from build123d import *

# Parameters (mm, degrees)
ESBO_O1_R                = 20
RESSALTO_EXTRUS_O1_DEPTH = 2
ESBO_O2_R                = 6
RESSALTO_EXTRUS_O2_DEPTH = 8
FILETE3_R                = 8
ESBO_O3_R                = 1.55
CORTE_EXTRUS_O1_DEPTH    = 30.393876913
PADR_OCIRCULAR1_COUNT    = 4
ESBO_O5_R                = 3.75
CORTE_EXTRUS_O2_DEPTH    = 6
PADR_OCIRCULAR2_COUNT    = 4


with BuildPart() as part:
    # Esboço1 → Ressalto-extrusão1 (new body)
    with BuildSketch(Plane.XY):
        Circle(ESBO_O1_R)
    extrude(amount=RESSALTO_EXTRUS_O1_DEPTH)

    # Esboço2 → Ressalto-extrusão2 (add)
    with BuildSketch(Plane.XY.offset(2)):
        Circle(ESBO_O2_R)
        with BuildLine():
            Line((-2.258317958, 2.05), (2.258317958, 2.05))
            ThreePointArc((2.258317958, 2.05), (0, -3.05), (-2.258317958, 2.05))
        make_face(mode=Mode.SUBTRACT)
    extrude(amount=RESSALTO_EXTRUS_O2_DEPTH)

    # Filete3
    filete3_edges = [part.edges().sort_by_distance(p)[0] for p in [
        (-6, 0, 2),
    ]]
    fillet(filete3_edges, radius=FILETE3_R - 0.0001)  # a hair under: the kernel refuses the full size

    # Esboço3 → Corte-extrusão1 (cut, through all)
    with BuildSketch(Plane.XY.offset(2)):
        with Locations((0, -12.5)):
            Circle(ESBO_O3_R)
    corte_extrus_o1 = extrude(amount=-CORTE_EXTRUS_O1_DEPTH, mode=Mode.SUBTRACT)

    # PadrãoCircular1: Corte-extrusão1 ×4 about axis
    padr_ocircular1_axis = Axis((0, 0, 0), (0, 0, 1))
    for i in range(1, PADR_OCIRCULAR1_COUNT):
        add(corte_extrus_o1.rotate(padr_ocircular1_axis, i * 360 / PADR_OCIRCULAR1_COUNT), mode=Mode.SUBTRACT)

    # Esboço5 → Corte-extrusão2 (cut)
    with BuildSketch(Plane.XY.offset(2)):
        with Locations((12.5, 0)):
            Circle(ESBO_O5_R)
    corte_extrus_o2 = extrude(amount=CORTE_EXTRUS_O2_DEPTH, mode=Mode.SUBTRACT)

    # PadrãoCircular2: Corte-extrusão2 ×4 about axis
    padr_ocircular2_axis = Axis((0, 0, 0), (0, 0, 1))
    for i in range(1, PADR_OCIRCULAR2_COUNT):
        add(corte_extrus_o2.rotate(padr_ocircular2_axis, i * 360 / PADR_OCIRCULAR2_COUNT), mode=Mode.SUBTRACT)


solid = part.part
Check sheet for the modelled part. Datum: model origin and axes. Units: mm. A direction names the side the tool comes from. Give positions to 0.01 mm unless a question says otherwise; leave off trailing zeros. Write each loop counter-clockwise with the first axis right and the second up, starting at its lowest first coordinate (ties: lowest second). Pieces come first, ordered by that corner, then holes. Notation, with made-up numbers: (-19.75, -23.75) -> (3.25, -23.75) arc R9 ccw to (3.25, -19.75) -> close; hole circle Ø8 at (66.25, 81.25). An arc over 180 degrees is marked (long way). One line per item, written item: value. Start each with the question number.
Item 1: Gauge pin test, flat ends, axial feed: pin 1 (10 mm diameter, centred on x = 12.5, y = 0, fed in from -Z); pin 2 (8.5 mm diameter, centred on x = 0, y = -12.5, fed in from +Z); pin 3 (2.5 mm diameter, centred on x = 1, z = 7.5, fed in from -Y); pin 4 (6 mm diameter, centred on x = 0, y = 12.5, fed in from +Z). Record the tip position at first contact, or that the pin passes through.
Item 2: Section check A-A on x = 0. State how many separate pieces and enclosed holes the cut face has, then the cut area to 3 significant figures.
Item 3: Draft check along X on faces 1 (the cylindrical face through (-14.013, 0.336, 1.014)), 2 (the cylindrical face through (-4.336, -19.524, 0.986)), 3 (the flat face through (0, 0, 0)). Enter one of: +X half, -X half, draft (parallel to the pull), parting line (faces both ways), or undercut.
Item 4: Material ranges on probe 1 along Y at (x, z) = (0, 1.3); probe 2 along Y at (x, z) = (0, 3.45); probe 3 along X at (y, z) = (0, 3), recorded low to high. Write a range as from..to.
Item 5: Section check C-C on z = 0.5. Record the cut outline in (x, y).
Item 6: Section check D-D on z = 5.75. Record the cut outline in (x, y).
Item 7: Tool access check on faces 4 (the cylindrical face through (-0.336, -14.013, 1.014)), 5 (the flat face through (0, 0, 2)). Record the directions out of +Z, -Z, +X, -X, +Y, -Y that give a thin tool (end or side, any length) a straight path to the whole face; none if there is none.
Results list:
1. pin 1: z = 0
1. pin 2: z = 4.44
1. pin 3: y = -6.88
1. pin 4: z = 2
2. separate pieces: 3
2. enclosed holes: 0
2. area: 144 mm²
3. face 1: undercut
3. face 2: parting line
3. face 3: draft
4. probe 1: -20..-14.05, -10.95..10.95, 14.05..20
4. probe 2: -8.75..-3.05, 2.05..8.75
4. probe 3: -8.75..-3.05, 3.05..8.75
5. outline: circle Ø40 at (0, 0); hole circle Ø3.1 at (-12.5, 0); hole circle Ø3.1 at (0, -12.5); hole circle Ø3.1 at (0, 12.5); hole circle Ø3.1 at (12.5, 0)
6. outline: circle Ø14.44 at (0, 0); hole (-2.26, 2.05) arc R3.05 ccw (long way) to (2.26, 2.05) -> close
7. face 4: +Z, -Z
7. face 5: +Z
